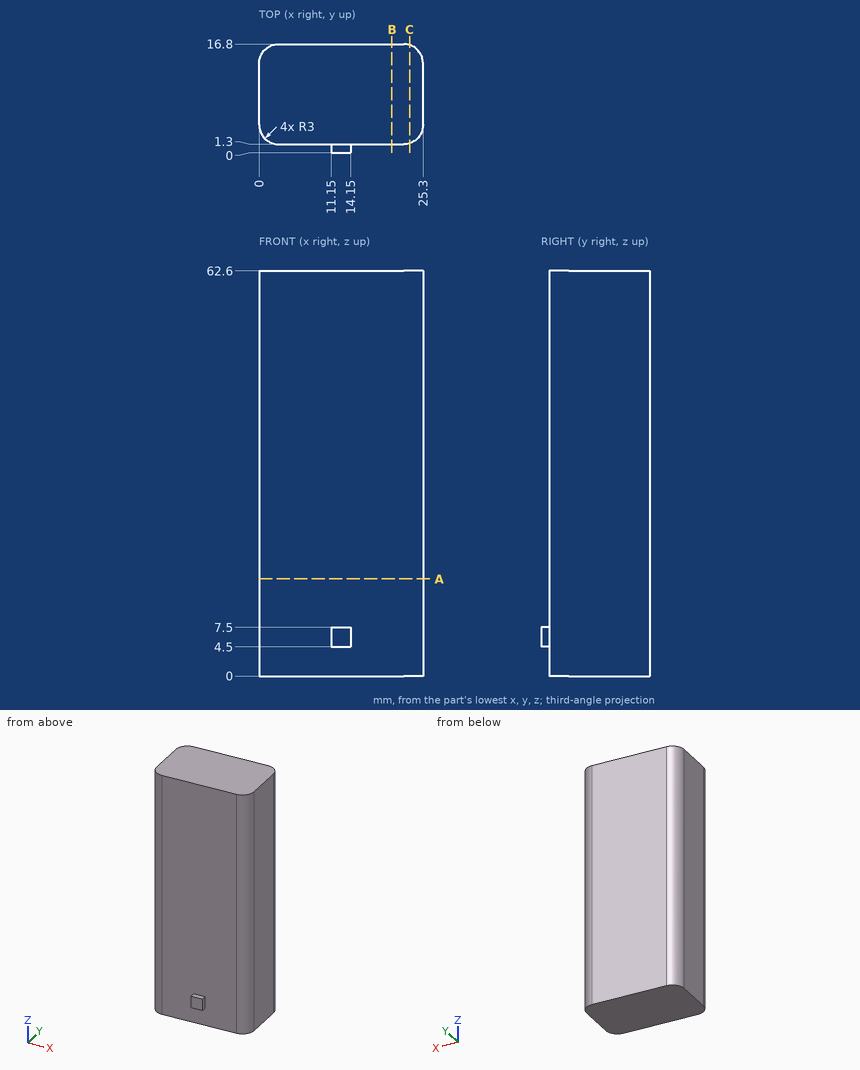
The drawing under review shows one solid part. Ordinate dimensions are in mm from its lowest x, y, z. Round coordinates to 2 decimals unless told otherwise and drop trailing zeros. Write each loop counter-clockwise with the first axis right and the second up, starting at its lowest first coordinate (ties: lowest second). Pieces come first, ordered by that corner, then holes. Notation, with made-up numbers: (60.25, 5.25) - (79.25, 5.25) arc R29 ccw to (79.25, 35.25) - close; hole circle Ø2 at (0.5, -11.75). An arc over 180 degrees is marked (long way). Write each question's results on one line, items separated by ' | '.
Item 1: For pin 1 (1 mm diameter, centred on y = 0.5, z = 6, fed in from -X); pin 2 (6 mm diameter, centred on x = 8, z = 23.5, fed in from -Y), all flat-tipped, find the tip position at first contact; note any pin that passes through.
Calculated:
pin 1: stops at x = 11.15 | pin 2: stops at y = 1.3
Item 2: Take a section at A-A on z = 15. State the section outline as (x, y) points.
Calculated:
outline: (0, 4.3) arc R3 ccw to (3, 1.3) - (22.3, 1.3) arc R3 ccw to (25.3, 4.3) - (25.3, 13.8) arc R3 ccw to (22.3, 16.8) - (3, 16.8) arc R3 ccw to (0, 13.8) - close
Item 3: Take a section at B-B on x = 20.5. State the section outline as (y, z) points.
Calculated:
outline: (1.3, 0) - (16.8, 0) - (16.8, 62.6) - (1.3, 62.6) - close
Item 4: Take a section at C-C on x = 23.25. State the section outline as (y, z) points, then the cut area to 3 significant figures.
Calculated:
outline: (1.45, 0) - (16.65, 0) - (16.65, 62.6) - (1.45, 62.6) - close | area: 951 mm^2
Item 5: To check wall thickness, follow line 1 along Y through (x, z) = (11.5, 37); line 2 along X through (y, z) = (15.25, 54). State the ranges of each line that lie inside material, in increasing order. Write a range as from..to.
Calculated:
line 1: y = 1.3..16.8 | line 2: x = 0.37..24.93
